Geometry check sheet. Reference: the model listing, model coordinates, mm. Round coordinates to 2 decimals unless told otherwise and drop trailing zeros. Write each loop counter-clockwise with the first axis right and the second up, starting at its lowest first coordinate (ties: lowest second). Pieces come first, ordered by that corner, then holes. Notation, with made-up numbers: M 11.25,54.25 L 31.25,54.25 A19 ccw 31.25,84.25 Z; hole C 35.5,-27 d8. An arc over 180 degrees is marked long. Put each result on its own line as item: value. Start each with the question number.
(1) Material ranges on probe 1 along X at (y, z) = (62.5, 2); probe 2 along Z at (x, y) = (-7, 68); probe 3 along Z at (x, y) = (-9, -59.5), recorded low to high.
(2) Gauge pin test, flat ends, axial feed: pin 1 (3.5 mm diameter, centred on x = 5, y = -15, fed in from -Z); pin 2 (1.7 mm diameter, centred on y = 20, z = 0, fed in from -X). Record the tip position at first contact, or that the pin passes through.
(3) Section check A-A on x = 5. Record the cut outline in (y, z), then the cut area to 3 significant figures.
(4) Section check C-C on y = 65.5. Record the cut outline in (x, z).
(5) Section check B-B on y = -5. Record the cut outline in (x, z), then the cut area to 3 significant figures.
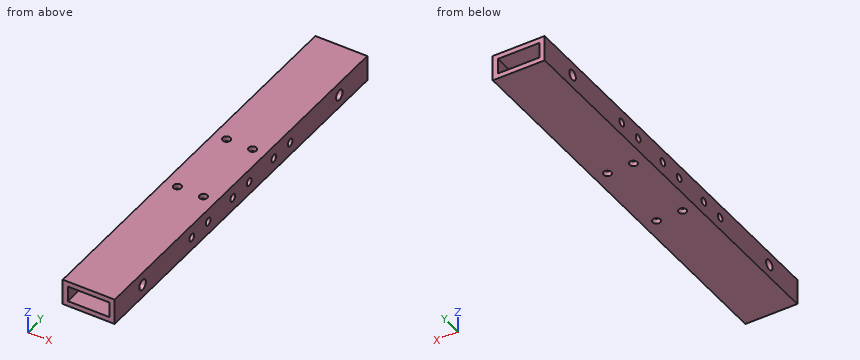
from build123d import *

# Parameters (mm, degrees)
SKETCH_1_W          = 20
SKETCH_1_H          = 10
SKETCH_1_W_2        = 16
SKETCH_1_H_2        = 6
EXTRUDE_1_DEPTH     = 77
SKETCH_2_R          = 1.45
SKETCH_2_R_2        = 2
CUT_EXTRUDE_1_DEPTH = 80.711981534
SKETCH_3_R          = 1.5
CUT_EXTRUDE_2_DEPTH = 79.287930104


with BuildPart() as part:
    # 草图1 → 凸台-拉伸1 (new, symmetric)
    with BuildSketch(Plane(origin=(0, 0, 0), x_dir=(1, 0, 0), z_dir=(0, 1, 0))):
        Rectangle(SKETCH_1_W, SKETCH_1_H)
        Rectangle(SKETCH_1_W_2, SKETCH_1_H_2, mode=Mode.SUBTRACT)
    extrude(amount=EXTRUDE_1_DEPTH, both=True)

    # 草图2 → 切除-拉伸1 (cut, through all)
    with BuildSketch(Plane(origin=(10, 0, 0), x_dir=(0, 0, -1), z_dir=(1, 0, 0))):
        with Locations((0, 5)):
            Circle(SKETCH_2_R)
        with Locations((0, 20)):
            Circle(SKETCH_2_R)
        with Locations((0, 30)):
            Circle(SKETCH_2_R)
        with Locations((0, -30)):
            Circle(SKETCH_2_R)
        with Locations((0, -20)):
            Circle(SKETCH_2_R)
        with Locations((0, -5)):
            Circle(SKETCH_2_R)
        with Locations((0, 60)):
            Circle(SKETCH_2_R_2)
        with Locations((0, -60)):
            Circle(SKETCH_2_R_2)
    extrude(amount=-CUT_EXTRUDE_1_DEPTH, mode=Mode.SUBTRACT)

    # 草图3 → 切除-拉伸2 (cut, through all)
    with BuildSketch(Plane(origin=(0, 0, -5), x_dir=(-1, 0, 0), z_dir=(0, 0, -1))):
        with Locations((5, -15)):
            Circle(SKETCH_3_R)
        with Locations((-5, -15)):
            Circle(SKETCH_3_R)
        with Locations((5, 15)):
            Circle(SKETCH_3_R)
        with Locations((-5, 15)):
            Circle(SKETCH_3_R)
    extrude(amount=-CUT_EXTRUDE_2_DEPTH, mode=Mode.SUBTRACT)


solid = part.part
Answers follow:
1. probe 1: x = -10 to -8, 8 to 10
1. probe 2: z = -5 to -3, 3 to 5
1. probe 3: z = -5 to -1.94, 1.94 to 5
2. pin 1: stops at z = -5
2. pin 2: passes through
3. outline: M -77,-5 L -16.5,-5 L -16.5,-3 L -77,-3 Z; M -77,3 L -16.5,3 L -16.5,5 L -77,5 Z; M -13.5,-5 L 13.5,-5 L 13.5,-3 L -13.5,-3 Z; M -13.5,3 L 13.5,3 L 13.5,5 L -13.5,5 Z; M 16.5,-5 L 77,-5 L 77,-3 L 16.5,-3 Z; M 16.5,3 L 77,3 L 77,5 L 16.5,5 Z
3. area: 592 mm^2
4. outline: M -10,-5 L 10,-5 L 10,5 L -10,5 Z; hole M -8,-3 L 8,-3 L 8,3 L -8,3 Z
5. outline: M -10,-5 L 10,-5 L 10,-1.45 L 8,-1.45 L 8,-3 L -8,-3 L -8,-1.45 L -10,-1.45 Z; M -10,1.45 L -8,1.45 L -8,3 L 8,3 L 8,1.45 L 10,1.45 L 10,5 L -10,5 Z
5. area: 92.4 mm^2
